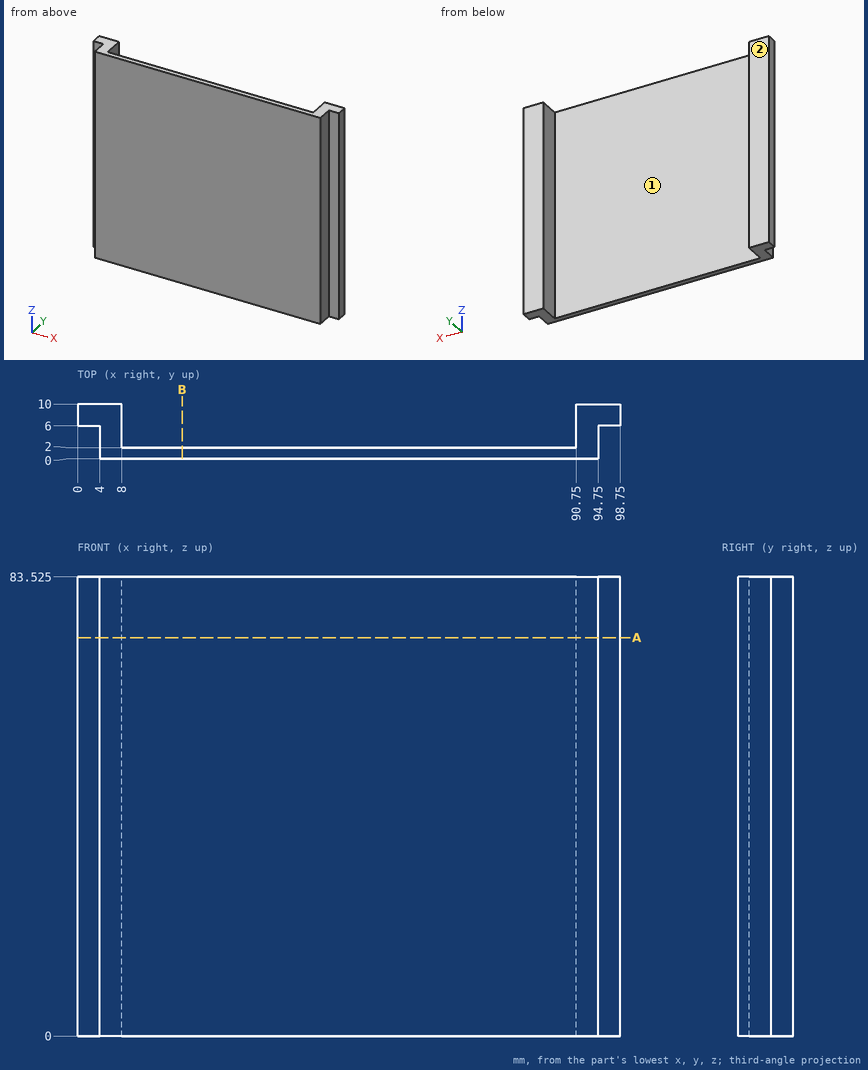
Study the drawing (mm; zero at the part's minimum x, y, z) and answer. A direction names the side the tool comes from. Give positions to 0.01 mm unless a question says otherwise; leave off trailing zeros. Write each loop counter-clockwise with the first axis right and the second up, starting at its lowest first coordinate (ties: lowest second). Pieces come first, ordered by that corner, then holes. Notation, with made-up numbers: (7.5, -32) -> (22.5, -32) arc R19 ccw to (22.5, -11) -> close; hole circle Ø10 at (59.25, 75). An arc over 180 degrees is marked (long way). Answer as a JSON object with one key per item and string values. Group by question number.
1) Each of these flat-tipped pins is pushed along its axis until it touches: P1, Ø2, axis at x = 2, z = 40, coming from the -Y side; P2, Ø3, axis at x = 32.5, z = 72.5, coming from the +Y side. Where does it stop, or does it pass through?
2) Find section A-A (z = 72.5). Write down the section's boundary in (x, y).
3) Consider L1, parallel to X at y = 7.25, z = 30; L2, parallel to X at y = 2.5, z = 62.5; L3, parallel to Y at x = 72, z = 14.5. Determine where each line is inside the solid, lowest interval first. Write a range as from..to.
4) A tool of negligible diameter and unlimited length cuts with its end or side. For the marked faces 1 and 2, from which of +Z, -Z, +X, -X, +Y, -Y can it reach the whole face along a straight path? Write none if from no direction.
5) Find section B-B (x = 19). Write down the section's boundary in (y, z) (3 decimals).
Values follow:
{
 "1": {"P1": "stops at y = 6", "P2": "stops at y = 2"},
 "2": {"outline": "(0, 6) -> (4, 6) -> (4, 0) -> (94.75, 0) -> (94.75, 6) -> (98.75, 6) -> (98.75, 10) -> (90.75, 10) -> (90.75, 2) -> (8, 2) -> (8, 10) -> (0, 10) -> close"},
 "3": {"L1": "x = 0..8, 90.75..98.75", "L2": "x = 4..8, 90.75..94.75", "L3": "y = 0..2"},
 "4": {"face 1": "+Z, -Z, +Y", "face 2": "+Z, -Z, +X, -X, +Y"},
 "5": {"outline": "(0, 0) -> (2, 0) -> (2, 83.525) -> (0, 83.525) -> close"}
}
